Verification items for the finished model (mm, model axes). A direction names the side the tool comes from. Give positions to 0.01 mm unless a question says otherwise; leave off trailing zeros. Order: outer loops, then holes, each group sorted by start corner. A loop starts at its lowest first (then second) coordinate and runs counter-clockwise, first axis right, second up.
(1) Mould release check, pull along X, two halves, no side actions. Record for faces 5 (the face through (33.797, 5.916, -47.627)), 6 (the face through (5.756, 5.916, -8.574)), 7 (the face through (47.508, 5.916, -53.116)), 8 (the face through (11.373, 5.916, -12.786)): pulls with the +X half, pulls with the -X half, needs draft (parallel to the pull), parting line crosses it, or undercut.
(2) Sectioned sample at C-C on z = -5. Record the cut outline in (x, y).
(3) Sectioned sample at B-B on x = 24. Record the cut outline in (y, z).
(4) Scan lines: L1, parallel to Z at x = 14, y = 7.75; L2, parallel to Z at x = 8, y = 3.5; L3, parallel to Z at x = 7, y = 3.5. Record each from-to range of solid material in increasing order.
(5) Gauge pin test, flat ends, axial feed: pin 1 (4 mm diameter, centred on x = 38.5, y = 7, fed in from +Z); pin 2 (3.5 mm diameter, centred on y = 4, z = -3.5, fed in from -X); pin 3 (1.1 mm diameter, centred on y = 6, z = 1, fed in from -X). Record the tip position at first contact, or that the pin passes through.
(6) Access from +Z, -Z, +X, -X, +Y, -Y to the whole of each face (thin tool, end or side, straight path). Record for faces 1 (the face through (13.74, 6, -26)), 2 (the face through (3.327, 5.916, -39.327)), 3 (the face through (18, 6, -49.672)), 4 (the face through (13, 4, 2)).
(7) Sectioned sample at A-A on x = 5. Record the cut outline in (y, z), plus the area to 3 significant figures.
```python
from build123d import *

# Parameters (mm, degrees)
SKETCH1_R           = 2.25
BOSS_EXTRUDE1_DEPTH = 12
SKETCH2_W           = 8
SKETCH2_H           = 4
BOSS_EXTRUDE2_DEPTH = 4
CUT_EXTRUDE1_DEPTH  = 6
CUT_EXTRUDE2_DEPTH  = 13
FILLET1_R           = 0.25


with BuildPart() as part:
    # Sketch1 → Boss-Extrude1 (new body)
    with BuildSketch(Plane(origin=(0, 0, 0), x_dir=(1, 0, 0), z_dir=(0, 1, 0))):
        Polygon((0, 0), (0, 8.7351098), (1.053451476, 9.722150715), (2.345646332, 7.07227283), (9.090891126, 10.042655859), (13.740010344, 15.630633236), (13.740010344, 36.934074296), (9.953212595, 40.720872045), (7.064267003, 40.720872045), (-0.809396561, 37.783381234), (-0.809396561, 45.604675912), (3.258374293, 49.672446766), (32.361506358, 49.672446766), (35.384723628, 45.363574987), (44.093237241, 55.930159978), (50.92671808, 50.298306266), (47.211057141, 20.639259086), (31.116613422, 0), align=None)
        with Locations((31.116613422, 39.692144587)):
            Circle(SKETCH1_R, mode=Mode.SUBTRACT)
    extrude(amount=BOSS_EXTRUDE1_DEPTH)

    # Sketch2 → Boss-Extrude2 (add)
    with BuildSketch(Plane.XY):
        with Locations((12, 6)):
            Rectangle(SKETCH2_W, SKETCH2_H)
    extrude(amount=BOSS_EXTRUDE2_DEPTH)

    # Sketch3 → Cut-Extrude1 (cut)
    with BuildSketch(Plane(origin=(0, 8, 0), x_dir=(1, 0, 0), z_dir=(0, 1, 0))):
        with BuildLine():
            Line((8, 0), (12, 0))
            ThreePointArc((12, 0), (12.353553391, -0.146446609), (12.5, -0.5))
            Line((12.5, -0.5), (12.5, -1.5))
            ThreePointArc((12.5, -1.5), (12.353553391, -1.853553391), (12, -2))
            Line((12, -2), (8, -2))
            Line((8, -2), (8, 0))
        make_face()
        with BuildLine():
            Line((14, -4), (16, -4))
            Line((16, -4), (16, -2))
            ThreePointArc((16, -2), (15.414213562, -3.414213562), (14, -4))
        make_face()
    extrude(amount=-CUT_EXTRUDE1_DEPTH, mode=Mode.SUBTRACT)

    # Sketch4 → Cut-Extrude2 (cut, through all)
    with BuildSketch(Plane(origin=(0, 12, 0), x_dir=(1, 0, 0), z_dir=(0, 1, 0))):
        Polygon((0, 0), (0, 1.364035653), (1.364035653, 0), align=None)
    extrude(amount=-CUT_EXTRUDE2_DEPTH, mode=Mode.SUBTRACT)

    # Fillet1
    fillet1_edges = [part.edges().sort_by_distance(p)[0] for p in [
        (1.364035653, 6, 0),
        (0, 6, -1.364035653),
        (0, 6, -8.7351098),
        (1.053451476, 6, -9.722150715),
        (2.345646332, 6, -7.07227283),
        (9.090891126, 6, -10.042655859),
        (13.740010344, 6, -15.630633236),
        (13.740010344, 6, -36.934074296),
        (9.953212595, 6, -40.720872045),
        (7.064267003, 6, -40.720872045),
        (-0.809396561, 6, -37.783381234),
        (-0.809396561, 6, -45.604675912),
        (3.258374293, 6, -49.672446766),
        (32.361506358, 6, -49.672446766),
        (35.384723628, 6, -45.363574987),
        (44.093237241, 6, -55.930159978),
        (50.92671808, 6, -50.298306266),
        (47.211057141, 6, -20.639259086),
        (31.116613422, 6, 0),
    ]]
    fillet(fillet1_edges, radius=FILLET1_R)


solid = part.part
```
Ans:
1. face 5: undercut
1. face 6: undercut
1. face 7: pulls with the +X half
1. face 8: pulls with the -X half
2. outline: (0, 0) - (35.02, 0) - (35.02, 12) - (0, 12) - close
3. outline: (0, -49.67) - (12, -49.67) - (12, 0) - (0, 0) - close
4. L1: z = -49.67 to 4
4. L2: z = -49.67 to -40.72, -9.56 to 0
4. L3: z = -49.67 to -40.7, -9.12 to 0
5. pin 1: stops at z = -6.9
5. pin 2: stops at x = 0
5. pin 3: stops at x = 12.5
6. face 1: -X, +Y, -Y
6. face 2: +Y, -Y
6. face 3: -Z, -X, +Y, -Y
6. face 4: +Z, +X, -X, -Y
7. outline: (0, -49.67) - (12, -49.67) - (12, -39.95) - (0, -39.95) - close; (0, -8.24) - (12, -8.24) - (12, 0) - (0, 0) - close
7. area: 216 mm2
